```python
from build123d import *

# Parameters (mm, degrees)
F0_R     = 11.125
F1_DEPTH = 7


with BuildPart() as f1:
    # F0 (on Front) → F1 (new body)
    with BuildSketch(Plane.XZ):
        with BuildLine():
            ThreePointArc((-10.632867, 8.318182), (0, 16.5), (10.632867, 8.318182))
            ThreePointArc((10.632867, 8.318182), (13.056476, 12.097679), (14.888415, 16.196762))
            ThreePointArc((14.888415, 16.196762), (16.6416, 27.339077), (14.153044, 38.340529))
            ThreePointArc((14.153044, 38.340529), (0, 25.75), (-14.153044, 38.340529))
            ThreePointArc((-14.153044, 38.340529), (-16.65233, 27.336563), (-14.895904, 16.189874))
            ThreePointArc((-14.895904, 16.189874), (-13.06061, 12.093603), (-10.632867, 8.318182))
        make_face()
        with BuildLine():
            ThreePointArc((-12.52019, 5.049242), (-11.691343, 6.75), (-10.632867, 8.318182))
            ThreePointArc((-10.632867, 8.318182), (-13.06061, 12.093603), (-14.895904, 16.189874))
            ThreePointArc((-14.895904, 16.189874), (-19.055102, 10.995594), (-21.471015, 4.795365))
            ThreePointArc((-21.471015, 4.795365), (-17.005135, 5.2584), (-12.52019, 5.049242))
        make_face()
        with BuildLine():
            ThreePointArc((-6.57289, -20.995169), (-3.943063, -17.357621), (-1.887323, -13.367423))
            ThreePointArc((-1.887323, -13.367423), (-14.289419, -8.25), (-12.52019, 5.049242))
            ThreePointArc((-12.52019, 5.049242), (-17.005135, 5.2584), (-21.471015, 4.795365))
            ThreePointArc((-21.471015, 4.795365), (-31.997135, 0.74251), (-40.280394, -6.913369))
            ThreePointArc((-40.280394, -6.913369), (-26.808348, -8.095723), (-20.391016, -20))
            ThreePointArc((-20.391016, -20), (-21.905588, -26.393073), (-26.12735, -31.42716))
            ThreePointArc((-26.12735, -31.42716), (-15.347993, -28.089622), (-6.57289, -20.995169))
        make_face()
        with BuildLine():
            ThreePointArc((6.582599, -20.992127), (3.948659, -17.356079), (1.887323, -13.367423))
            ThreePointArc((1.887323, -13.367423), (0, -13.5), (-1.887323, -13.367423))
            ThreePointArc((-1.887323, -13.367423), (-3.943063, -17.357621), (-6.57289, -20.995169))
            ThreePointArc((-6.57289, -20.995169), (0.005087, -21.999999), (6.582599, -20.992127))
        make_face()
        with BuildLine():
            ThreePointArc((21.468795, 4.805294), (17.003672, 5.264018), (12.52019, 5.049242))
            ThreePointArc((12.52019, 5.049242), (14.289419, -8.25), (1.887323, -13.367423))
            ThreePointArc((1.887323, -13.367423), (3.948659, -17.356079), (6.582599, -20.992127))
            ThreePointArc((6.582599, -20.992127), (15.355535, -28.081587), (26.12735, -31.42716))
            ThreePointArc((26.12735, -31.42716), (22.300154, -12.875), (40.280394, -6.913369))
            ThreePointArc((40.280394, -6.913369), (32.000323, 0.753059), (21.468795, 4.805294))
        make_face()
        with BuildLine():
            ThreePointArc((12.52019, 5.049242), (13.252784, 2.571715), (13.5, 0))
            ThreePointArc((13.5, 0), (10.19139, -8.853562), (1.887323, -13.367423))
            ThreePointArc((1.887323, -13.367423), (14.289419, -8.25), (12.52019, 5.049242))
        make_face()
        with BuildLine():
            ThreePointArc((1.887323, -13.367423), (10.19139, -8.853562), (13.5, 0))
            ThreePointArc((13.5, 0), (13.252784, 2.571715), (12.52019, 5.049242))
            ThreePointArc((12.52019, 5.049242), (11.691343, 6.75), (10.632867, 8.318182))
            ThreePointArc((10.632867, 8.318182), (0, 13.5), (-10.632867, 8.318182))
            ThreePointArc((-10.632867, 8.318182), (-11.691343, 6.75), (-12.52019, 5.049242))
            ThreePointArc((-12.52019, 5.049242), (-11.691343, -6.75), (-1.887323, -13.367423))
            ThreePointArc((-1.887323, -13.367423), (0, -13.5), (1.887323, -13.367423))
        make_face()
        Circle(F0_R, mode=Mode.SUBTRACT)
        with BuildLine():
            ThreePointArc((-12.52019, 5.049242), (-14.289419, -8.25), (-1.887323, -13.367423))
            ThreePointArc((-1.887323, -13.367423), (-11.691343, -6.75), (-12.52019, 5.049242))
        make_face()
        with BuildLine():
            ThreePointArc((-10.632867, 8.318182), (0, 13.5), (10.632867, 8.318182))
            ThreePointArc((10.632867, 8.318182), (0, 16.5), (-10.632867, 8.318182))
        make_face()
        with BuildLine():
            ThreePointArc((-14.153044, 38.340529), (0, 25.75), (14.153044, 38.340529))
            ThreePointArc((14.153044, 38.340529), (14.22574, 39.168849), (14.25, 40))
            ThreePointArc((14.25, 40), (-0.831151, 54.22574), (-14.153044, 38.340529))
        make_face()
        with Locations((0, 40)):
            Circle(F0_R, mode=Mode.SUBTRACT)
        with BuildLine():
            ThreePointArc((10.632867, 8.318182), (11.691343, 6.75), (12.52019, 5.049242))
            ThreePointArc((12.52019, 5.049242), (17.003672, 5.264018), (21.468795, 4.805294))
            ThreePointArc((21.468795, 4.805294), (19.050015, 11.004405), (14.888415, 16.196762))
            ThreePointArc((14.888415, 16.196762), (13.056476, 12.097679), (10.632867, 8.318182))
        make_face()
        with BuildLine():
            ThreePointArc((48.891016, -20), (46.545293, -12.167332), (40.280394, -6.913369))
            ThreePointArc((40.280394, -6.913369), (22.300154, -12.875), (26.12735, -31.42716))
            ThreePointArc((26.12735, -31.42716), (41.034089, -32.735428), (48.891016, -20))
        make_face()
        with Locations((34.641016, -20)):
            Circle(F0_R, mode=Mode.SUBTRACT)
        with BuildLine():
            ThreePointArc((-40.280394, -6.913369), (-46.981878, -27.125), (-26.12735, -31.42716))
            ThreePointArc((-26.12735, -31.42716), (-21.905588, -26.393073), (-20.391016, -20))
            ThreePointArc((-20.391016, -20), (-26.808348, -8.095723), (-40.280394, -6.913369))
        make_face()
        with Locations((-34.641016, -20)):
            Circle(F0_R, mode=Mode.SUBTRACT)
    extrude(amount=F1_DEPTH)


solid = f1.part
```
Can you work these out from the model? Positions are in its coordinate system, mm. A direction names the side the tool comes from. Give positions to 0.01 mm unless a question says otherwise; leave off trailing zeros. Write each loop counter-clockwise with the first axis right and the second up, starting at its lowest first coordinate (ties: lowest second). Pieces come first, ordered by that corner, then holes. Notation, with made-up numbers: (-1.5, 40.25) -> (37.5, 40.25) arc R29 cw to (37.5, 74.25) -> close; hole circle Ø11 at (62.5, 30.25). An arc over 180 degrees is marked (long way). One line per item, written item: value.
Q1. Imagine slicing it at D-D on z = 22.5. Please give me the cut outline in (x, y), and give its area (3 significant figures).
Results found:
outline: (-16.42, -7) -> (16.41, -7) -> (16.41, 0) -> (-16.42, 0) -> close
area: 230 mm^2
Q2. For P1, Ø1, axis at x = 7.5, z = 34.5, coming from the +Y side; P2, Ø2, axis at y = -4, z = 3, coming from the +X side; P3, Ø1, axis at y = -6, z = 12.5, coming from the +X side; P4, Ø4, axis at x = -10.5, y = -6, coming from the -Z side, each with a flat end and sliding along its axis, tell me the tip position at first contact or that it passes through.
Results found:
P1: passes through
P2: stops at x = 29.8
P3: stops at x = 18.44
P4: stops at z = -26.36
Q3. We'd pull the mould along Z, two halves only. Please class faces 1 (the face through (0, -3, -22)), 2 (the face through (19.1, -3.45, 10.92)), 3 (the face through (-11, 0, 4)): +Z half, -Z half, draft (parallel to the pull), parting line (faces both ways), or undercut.
Results found:
face 1: -Z half
face 2: undercut
face 3: draft
Q4. Which directions (+Z, -Z, +X, -X, +Y, -Y) give clear straight access to the entire face, cutting with the end or side of a thin tool? Please do faces 4 (the face through (15.2, -3.5, -28)), 5 (the face through (-31.862, -3.451, 0.826)), 6 (the face through (-19.008, -3.451, 11.076)).
Results found:
face 4: -Z, +Y, -Y
face 5: +Z, -X, +Y, -Y
face 6: -X, +Y, -Y
Q5. Please list where these lines run through material, in increasing order: line 1 (Z direction, x = 0, y = -5) (3 decimals); line 2 (Z direction, x = -6.5, y = -3); line 3 (X direction, y = -4, z = -7). Write a range as [from, to].
Results found:
line 1: z = [-22, -11.125], [11.125, 28.875], [51.125, 54.25]
line 2: z = [-21.02, -9.03], [9.03, 30.97], [49.03, 52.68]
line 3: x = [-40.48, -8.65], [8.65, 40.48]
Q6. Imagine slicing it at C-C on y = -3.75. Please give me the cut outline in (x, z) (3 decimals), and give its area (3 significant figures).
Results found:
outline: (-40.28, -6.913) arc R14.25 ccw (long way) to (-26.127, -31.427) arc R29.904 ccw to (-6.573, -20.995) arc R22 ccw to (6.583, -20.992) arc R29.977 ccw to (26.127, -31.427) arc R14.25 ccw (long way) to (40.28, -6.913) arc R29.904 ccw to (21.469, 4.805) arc R22 ccw to (14.888, 16.197) arc R29.977 ccw to (14.153, 38.341) arc R14.25 ccw to (14.25, 40) arc R14.25 ccw (long way) to (-14.153, 38.341) arc R29.904 ccw to (-14.896, 16.19) arc R22 ccw to (-21.471, 4.795) arc R29.977 ccw to start; hole circle Ø22.25 at (-34.641, -20); hole circle Ø22.25 at (0, 0); hole circle Ø22.25 at (0, 40); hole circle Ø22.25 at (34.641, -20)
area: 2,830 mm^2
Q7. Imagine slicing it at B-B on z = 0. Please give me the cut outline in (x, y) (1 decimal), and give its area (3 significant figures).
Results found:
outline: (-33.1, -7) -> (-11.1, -7) -> (-11.1, 0) -> (-33.1, 0) -> close; (11.1, -7) -> (33.1, -7) -> (33.1, 0) -> (11.1, 0) -> close
area: 308 mm^2
Q8. Imagine slicing it at A-A on x = -38.5. Please give me the cut outline in (y, z).
Results found:
outline: (-7, -33.72) -> (0, -33.72) -> (0, -30.43) -> (-7, -30.43) -> close; (-7, -9.57) -> (0, -9.57) -> (0, -4.72) -> (-7, -4.72) -> close
